Model file for the job. Use its own axes, mm. A direction names the side the tool comes from. Give positions to 0.01 mm unless a question says otherwise; leave off trailing zeros. Write each loop counter-clockwise with the first axis right and the second up, starting at its lowest first coordinate (ties: lowest second). Pieces come first, ordered by that corner, then holes. Notation, with made-up numbers: (86.25, 88.25) - (102.25, 88.25) arc R17 ccw to (102.25, 111.25) - close; hole circle Ø6 at (-15, -21.75). An arc over 180 degrees is marked (long way). One line per item, written item: value. Start each with the question number.
(1) Cut at C-C, the plane z = 3.35. List the corners of the cut face in (x, y), and give its area (3 significant figures).
(2) Mould opens along Y. For faces 3 (the face through (-13.35, -14.14, 3.01)), 4 (the face through (-8.43, -1.94, 0.69)), 5 (the face through (-11, 10.406, 3)), 6 (the face through (-11, -7.169, 3)) say: pulls with the +Y half, pulls with the -Y half, needs draft (parallel to the pull), parting line crosses it, or undercut.
(3) Cut at B-B, the plane x = -10.9. List the corners of the cut face in (y, z), and give its area (3 significant figures).
(4) 3-axis set-ups, long thin cutter, end or side, ignore diameter. For faces 1 (the face through (-11, -10, 0)), 2 (the face through (-11.751, -2, 3)): which of +Z, -Z, +X, -X, +Y, -Y reach the whole face in a straight line?
(5) Cut at A-A, the plane y = 1.5. List the corners of the cut face in (x, z), and give its area (3 significant figures).
(6) Cut at D-D, the plane y = -11.25. List the corners of the cut face in (x, z), and give its area (3 significant figures).
(7) Probe L1, parallel to X at y = -1.5, z = 2.55; L2, parallel to Y at x = -10.9, z = 4.55; L3, parallel to Z at x = -11.75, y = -10.75. List the from-to ranges inside material, lowest first.
from build123d import *

# Parameters (mm, degrees)
F0_W        = 6
F0_H        = 25
F0_W_2      = 2
F0_H_2      = 10
F1_DEPTH    = 6
F2_T1_DEPTH = 36.5
F3_R        = 1.5


# Not quite as in the source:
# - a fillet or chamfer that OpenCascade refuses, or shapes differently, is made with other operations: its cross-section is extruded or revolved along the edge and cut away or added


with BuildPart() as f1:
    # F0 (on Top) → F1 (new body)
    with BuildSketch(Plane.XY):
        with Locations((-10.7731075219, -2.0936969668)):
            Rectangle(F0_W, F0_H)
        with Locations((-10.7510519922, -2.1686129086)):
            Rectangle(F0_W_2, F0_H_2, mode=Mode.SUBTRACT)
    extrude(amount=F1_DEPTH)

    # F2: fillet of radius 2.3 on 4 edges, made by hand

    # F2_s2 → F2_t1 (cut)
    with BuildSketch(Plane.XZ.offset(-16.1563030332)):
        with BuildLine():
            ThreePointArc((-13.7731075219, 3.7), (-13.0994531186, 5.3263455967), (-11.4731075219, 6))
            Line((-11.4731075219, 6), (-13.7731075219, 6))
            Line((-13.7731075219, 6), (-13.7731075219, 3.7))
        make_face()
        with BuildLine():
            ThreePointArc((-13.7731075219, 2.3), (-13.0994531186, 0.6736544033), (-11.4731075219, 0))
            Line((-11.4731075219, 0), (-13.7731075219, 0))
            Line((-13.7731075219, 0), (-13.7731075219, 2.3))
        make_face()
        with BuildLine():
            ThreePointArc((-7.7731075219, 3.7), (-8.4467619252, 5.3263455967), (-10.0731075219, 6))
            Line((-10.0731075219, 6), (-7.7731075219, 6))
            Line((-7.7731075219, 6), (-7.7731075219, 3.7))
        make_face()
        with BuildLine():
            ThreePointArc((-7.7731075219, 2.3), (-8.4467619252, 0.6736544033), (-10.0731075219, 0))
            Line((-10.0731075219, 0), (-7.7731075219, 0))
            Line((-7.7731075219, 0), (-7.7731075219, 2.3))
        make_face()
    extrude(amount=F2_T1_DEPTH, mode=Mode.SUBTRACT)

    # F3
    f3_edges = [f1.edges().sort_by_distance(p)[0] for p in [
        (-8.446762, 10.406303, 5.326346),
        (-10.773108, 10.406303, 6),
        (-13.099453, 10.406303, 5.326346),
        (-13.773108, 10.406303, 3),
        (-13.099453, 10.406303, 0.673654),
        (-8.446762, 10.406303, 0.673654),
        (-7.773108, 10.406303, 3),
        (-10.773108, 10.406303, 0),
        (-13.099453, -14.593697, 0.673654),
    ]]
    fillet(f3_edges, radius=F3_R)


solid = f1.part
Answers follow:
1. outline: (-13.77, -13.09) arc R1.5 ccw to (-12.27, -14.59) - (-9.27, -14.59) arc R1.5 ccw to (-7.77, -13.09) - (-7.77, 8.91) arc R1.5 ccw to (-9.27, 10.41) - (-12.27, 10.41) arc R1.5 ccw to (-13.77, 8.91) - close; hole (-11.75, -7.17) - (-9.75, -7.17) - (-9.75, 2.83) - (-11.75, 2.83) - close
1. area: 128 mm²
2. face 3: pulls with the -Y half
2. face 4: needs draft
2. face 5: pulls with the +Y half
2. face 6: undercut
3. outline: (-14.59, 1.5) arc R1.5 ccw to (-13.09, 0) - (-7.17, 0) - (-7.17, 6) - (-13.09, 6) arc R1.5 ccw to (-14.59, 4.5) - close; (2.83, 0) - (8.91, 0) arc R1.5 ccw to (10.41, 1.5) - (10.41, 4.5) arc R1.5 ccw to (8.91, 6) - (2.83, 6) - close
3. area: 88.1 mm²
4. face 1: -Z, +X, -X, +Y, -Y
4. face 2: +Z, -Z
5. outline: (-13.77, 2.3) arc R2.3 ccw to (-11.75, 0.02) - (-11.75, 5.98) arc R2.3 ccw to (-13.77, 3.7) - close; (-9.75, 0.02) arc R2.3 ccw to (-7.77, 2.3) - (-7.77, 3.7) arc R2.3 ccw to (-9.75, 5.98) - close
5. area: 19.5 mm²
6. outline: (-13.77, 2.3) arc R2.3 ccw to (-11.47, 0) - (-10.07, 0) arc R2.3 ccw to (-7.77, 2.3) - (-7.77, 3.7) arc R2.3 ccw to (-10.07, 6) - (-11.47, 6) arc R2.3 ccw to (-13.77, 3.7) - close
6. area: 31.5 mm²
7. L1: x = -13.77 to -11.75, -9.75 to -7.77
7. L2: y = -14.59 to -7.17, 2.83 to 10.41
7. L3: z = 0.02 to 5.98
